Geometry check sheet. Reference: the model listing, model coordinates, mm. Face numbers are marked on the shaded views. A direction names the side the tool comes from. Give positions to 0.01 mm unless a question says otherwise; leave off trailing zeros. Write each loop counter-clockwise with the first axis right and the second up, starting at its lowest first coordinate (ties: lowest second). Pieces come first, ordered by that corner, then holes. Notation, with made-up numbers: (76, 20.25) - (119, 20.25) arc R18 ccw to (119, 54.25) - close; hole circle Ø10 at (-38.75, 60). An arc over 180 degrees is marked (long way). One line per question, with ' | ' between items. Start each with the question number.
Q1. Section check D-D on y = -11.25. Record the boundary of the cut face in (x, z), and give its area (3 significant figures).
Q2. Section check C-C on z = 16. Record the boundary of the cut face in (x, y), and give its area (3 significant figures).
Q3. Release check for a two-part mould opening along X. For the marked faces 4, 5 and 6 record: +X half, -X half, draft (parallel to the pull), parting line (faces both ways), or undercut.
Q4. Thickness scan on L1, parallel to Z at x = 4, y = -1.5; L2, parallel to Y at x = 20, z = 6.5; L3, parallel to X at y = -13, z = 8.25. Record the ranges inside material, lowest first. Write a range as [from, to].
Q5. Set-up check for the marked faces 1, 2 and 3: record each of +Z, -Z, +X, -X, +Y, -Y from which the full face is reachable in a straight line by a thin tool's end or side.
Q6. Section check B-B on y = -1. Record the boundary of the cut face in (x, z) (3 decimals).
Q7. Gauge pin test, flat ends, axial feed: P1, Ø4, axis at x = -19.98, z = 18.25, coming from the -Y side; P2, Ø6, axis at y = -13.5, z = 3.5, coming from the -X side; P3, Ø3, axis at x = 1.5, y = -15, coming from the -Z side; P4, Ø1.5, axis at x = 1.5, y = -8.5, coming from the -Z side. Record the tip position at first contact, or that the pin passes through.
Q8. Section check A-A on z = 10.75. Record the boundary of the cut face in (x, y).
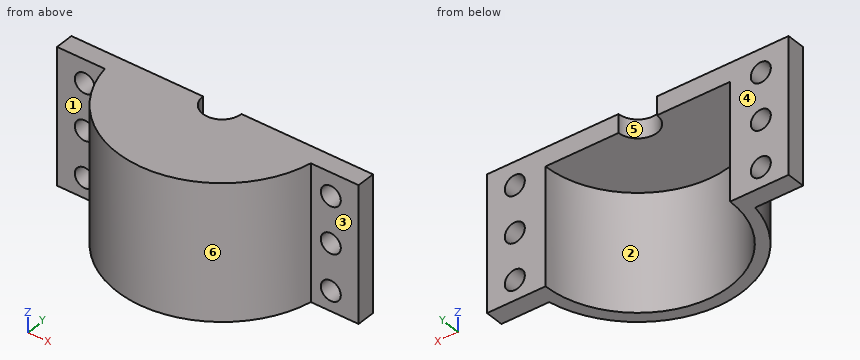
```python
from build123d import *

# Parameters (mm, degrees)
SALIENTE_EXTRUIR1_DEPTH = 19
SALIENTE_EXTRUIR2_DEPTH = 3
CROQUIS3_R              = 3.125
CORTAR_EXTRUIR1_DEPTH   = 3
CROQUIS4_W              = 7.766799469
CROQUIS4_H              = 3
SALIENTE_EXTRUIR3_DEPTH = 22
CROQUIS5_R              = 1.625
CORTAR_EXTRUIR2_DEPTH   = 4


with BuildPart() as part:
    # Croquis1 → Saliente-Extruir1 (new body)
    with BuildSketch(Plane.XY):
        with BuildLine():
            Line((17, 0), (15, 0))
            ThreePointArc((15, 0), (0, -15), (-15, 0))
            Line((-15, 0), (-17, 0))
            ThreePointArc((-17, 0), (0, -17), (17, 0))
        make_face()
    extrude(amount=SALIENTE_EXTRUIR1_DEPTH)

    # Croquis2 → Saliente-Extruir2 (add)
    with BuildSketch(Plane.XY.offset(19)):
        with BuildLine():
            Line((15, 0), (-15, 0))
            ThreePointArc((-15, 0), (0, -15), (15, 0))
        make_face()
        with BuildLine():
            ThreePointArc((15, 0), (0, -15), (-15, 0))
            Line((-15, 0), (-17, 0))
            ThreePointArc((-17, 0), (0, -17), (17, 0))
            Line((17, 0), (15, 0))
        make_face()
    extrude(amount=SALIENTE_EXTRUIR2_DEPTH)

    # Croquis3 → Cortar-Extruir1 (cut)
    with BuildSketch(Plane.XY.offset(22)):
        Circle(CROQUIS3_R)
    extrude(amount=-CORTAR_EXTRUIR1_DEPTH, mode=Mode.SUBTRACT)

    # Croquis4 → Saliente-Extruir3 (add)
    with BuildSketch(Plane.XY.offset(22)):
        with Locations((-20.616600266, -1.5)):
            Rectangle(CROQUIS4_W, CROQUIS4_H)
        with Locations((20.616600266, -1.5)):
            Rectangle(CROQUIS4_W, CROQUIS4_H)
    extrude(amount=-SALIENTE_EXTRUIR3_DEPTH)

    # Croquis5 → Cortar-Extruir2 (cut, through all)
    with BuildSketch(Plane.XZ.offset(3)):
        with Locations((-19.983200531, 3.25)):
            Circle(CROQUIS5_R)
        with Locations((-19.983200531, 10.75)):
            Circle(CROQUIS5_R)
        with Locations((-19.983200531, 18.25)):
            Circle(CROQUIS5_R)
        with Locations((19.983200531, 18.25)):
            Circle(CROQUIS5_R)
        with Locations((19.983200531, 10.75)):
            Circle(CROQUIS5_R)
        with Locations((19.983200531, 3.25)):
            Circle(CROQUIS5_R)
    extrude(amount=-CORTAR_EXTRUIR2_DEPTH, mode=Mode.SUBTRACT)


solid = part.part
```
Working result:
1) outline: (-12.75, 0) - (-9.92, 0) - (-9.92, 19) - (9.92, 19) - (9.92, 0) - (12.75, 0) - (12.75, 22) - (-12.75, 22) - close | area: 184 mm2
2) outline: (-24.5, -3) - (-16.73, -3) arc R17 ccw to (16.73, -3) - (24.5, -3) - (24.5, 0) - (15, 0) arc R15 cw to (-15, 0) - (-24.5, 0) - close | area: 146 mm2
3) face 4: draft | face 5: undercut | face 6: parting line
4) L1: z = [19, 22] | L2: y = [-3, 0] | L3: x = [-10.95, -7.48], [7.48, 10.95]
5) face 1: +Z, -Z, -X, -Y | face 2: -Z, +Y | face 3: +Z, -Z, +X, -Y
6) outline: (-24.5, 0) - (-14.967, 0) - (-14.967, 19) - (-2.961, 19) - (-2.961, 22) - (-24.5, 22) - close; (2.961, 19) - (14.967, 19) - (14.967, 0) - (24.5, 0) - (24.5, 22) - (2.961, 22) - close; hole circle Ø3.25 at (-19.983, 3.25); hole circle Ø3.25 at (-19.983, 10.75); hole circle Ø3.25 at (-19.983, 18.25); hole circle Ø3.25 at (19.983, 3.25); hole circle Ø3.25 at (19.983, 10.75); hole circle Ø3.25 at (19.983, 18.25)
7) P1: stops at y = -3 | P2: stops at x = -13.37 | P3: stops at z = 0 | P4: stops at z = 19
8) outline: (-24.5, -3) - (-21.61, -3) - (-21.61, 0) - (-24.5, 0) - close; (-18.36, -3) - (-16.73, -3) arc R17 ccw to (16.73, -3) - (18.36, -3) - (18.36, 0) - (15, 0) arc R15 cw to (-15, 0) - (-18.36, 0) - close; (21.61, -3) - (24.5, -3) - (24.5, 0) - (21.61, 0) - close
